Autodesk Inventor part; units mm, degrees
ref_plane "YZ Plane" through (0, 0, 0) normal (1, 0, 0) x (0, 1, 0)
ref_plane "XZ Plane" through (0, 0, 0) normal (0, 1, 0) x (-1, 0, 0)
ref_plane "XY Plane" through (0, 0, 0) normal (0, 0, 1) x (1, 0, 0)
sketch "Sketch1" plane through (0, 0, 0) normal (0, 1, 0) x (-1, 0, 0)
  line L0 (0, 0) -> (25, 0)
  line L1 (25, 0) -> (25, -50)
  line L2 (25, -50) -> (0, -50)
  line L3 (0, -50) -> (0, 0)
  dimension "d0" = 25
  dimension "d1" = 50
extrude "Extrusion1" add sketch "Sketch1" along normal blind 12
sketch "Sketch2" plane through (0, 12, 0) normal (0, 1, 0) x (1, 0, 0)
  circle A0 centre (-12.5, 15) radius 3.2
  circle A1 centre (-12.5, 35) radius 3.2
  line L0 (-25, 0) -> (0, 0)
  line L1 (0, 0) -> (0, 50)
  dimension "d4" = 6.4
  dimension "d5" = 20
  dimension "d6" = 15
  dimension "d7" = 12.5
extrude "Extrusion2" cut sketch "Sketch2" against normal through all
sketch "Sketch3" plane through (0, 12, 0) normal (0, 1, 0) x (1, 0, 0)
  circle A0 centre (-12.5, 15) radius 3.2
  circle A1 centre (-12.5, 15) radius 5.5
  circle A2 centre (-12.5, 35) radius 3.2
  circle A3 centre (-12.5, 35) radius 5.5
  point P0 (0, 0)
  dimension "d10" = 11
extrude "Extrusion3" cut sketch "Sketch3" against normal blind 6.8 contours A0 | A1 | A2 | A3
CAD build for the part. Positions are in the model's coordinates, mm. A direction names the side the tool comes from. Round coordinates to 2 decimals unless told otherwise and drop trailing zeros. Loops run counter-clockwise (first coordinate to the right, second up) from the corner with the lowest first, then second, coordinate; pieces in that order, holes last. Notation, with made-up numbers: (-2, 18) - (29, 18) arc R22 ccw to (29, 49) - close; hole circle Ø3 at (8.5, -38.5). An arc over 180 degrees is marked (long way). Return JSON: item names as keys, results as strings. Group by question number.
Q1. Tool access for faces 1 (the face through (-11.023, 2.636, -12.161)), 2 (the face through (-10.1, 5.2, -32.6)): list every direction of +Z, -Z, +X, -X, +Y, -Y with a clear straight run to the whole face (end or side of a thin tool).
Q2. Band-saw the part on A-A on x = -12.5. Give the cut face in (y, z).
Q3. Band-saw the part on C-C on y = 3.25. Give the cut face in (x, z), plus the area to 3 significant figures.
Q4. Band-saw the part on B-B on z = -15. Give the cut face in (x, y), plus the area to 3 significant figures.
Q5. Drill centre lines: line 1 along Z through (x, y) = (-12.5, 2.4); line 2 along Z through (x, y) = (-12.5, 9.25); line 3 along X through (y, z) = (9, -15). Where is each one in solid material? Low to high. Write a range as [from, to].
Q6. Flat gauge pins, fed straight in: pin 1 Ø6 at (x, z) = (-12.5, -15) entering from -Y; pin 2 Ø12 at (x, z) = (-17, -24) entering from -Y; pin 3 Ø6.5 at (x, z) = (-12.5, -15) entering from +Y. Where does each tip first touch, or does it go through?
Q7. Two-plate mould, pull along X, no slides. Class faces 3 (the face through (-12.917, 2.636, -38.173)), 4 (the face through (-12, 12, -25)), 5 (the face through (-25, 6, -25)): +X half, -X half, draft (parallel to the pull), parting line (faces both ways), or undercut.
Q8. Band-saw the part on D-D on y = 7. Give the cut face in (x, z), plus the area to 3 significant figures.
Solutions:
{
 "1": {"face 1": "+Y, -Y", "face 2": "+Y"},
 "2": {"outline": "(0, -50) - (12, -50) - (12, -40.5) - (5.2, -40.5) - (5.2, -38.2) - (0, -38.2) - close; (0, -31.8) - (5.2, -31.8) - (5.2, -29.5) - (12, -29.5) - (12, -20.5) - (5.2, -20.5) - (5.2, -18.2) - (0, -18.2) - close; (0, -11.8) - (5.2, -11.8) - (5.2, -9.5) - (12, -9.5) - (12, 0) - (0, 0) - close"},
 "3": {"outline": "(-25, -50) - (0, -50) - (0, 0) - (-25, 0) - close; hole circle Ø6.4 at (-12.5, -35); hole circle Ø6.4 at (-12.5, -15)", "area": "1,190 mm^2"},
 "4": {"outline": "(-25, 0) - (-15.7, 0) - (-15.7, 5.2) - (-18, 5.2) - (-18, 12) - (-25, 12) - close; (-9.3, 0) - (0, 0) - (0, 12) - (-7, 12) - (-7, 5.2) - (-9.3, 5.2) - close", "area": "192 mm^2"},
 "5": {"line 1": "z = [-50, -38.2], [-31.8, -18.2], [-11.8, 0]", "line 2": "z = [-50, -40.5], [-29.5, -20.5], [-9.5, 0]", "line 3": "x = [-25, -18], [-7, 0]"},
 "6": {"pin 1": "passes through", "pin 2": "stops at y = 0", "pin 3": "stops at y = 5.2"},
 "7": {"face 3": "undercut", "face 4": "draft", "face 5": "-X half"},
 "8": {"outline": "(-25, -50) - (0, -50) - (0, 0) - (-25, 0) - close; hole circle Ø11 at (-12.5, -35); hole circle Ø11 at (-12.5, -15)", "area": "1,060 mm^2"}
}
